Can you work these out from the model? Positions are in its coordinate system, mm. A direction names the side the tool comes from. Round coordinates to 2 decimals unless told otherwise and drop trailing zeros. Order: outer loops, then holes, each group sorted by start corner. A loop starts at its lowest first (then second) coordinate and runs counter-clockwise, first axis right, second up. Notation, with made-up numbers: (-3, 26.25) -> (10, 26.25) arc R30 cw to (10, 52.25) -> close; hole circle Ø10 at (-11, 21). An arc over 180 degrees is marked (long way). Use a Markdown table: item, result. Add a question column.
Q1. If we section it at A-A on x = 45: List the corners of the cut face in (y, z) for me.
Q2. I need wall thicknesses on line 1 along X through (y, z) = (73, 5.25); line 2 along Y through (x, z) = (161.5, 5); line 3 along Y through (x, z) = (30.5, 9.75). Which ranges of each line are inside material? Lowest first, please. Write a range as [from, to].
Q3. If we section it at B-B on z = 7: Give the number of separate pieces and of enclosed holes in the cut face, plus the area to 3 significant figures.
Q4. For faces 1 (the face through (245.316, 106, 5)), 2 (the face through (39, 37.988, 5)), 3 (the face through (260, 257.988, 5)), which set-ups out of +Z, -Z, +X, -X, +Y, -Y let a thin tool reach every point of the face, with its end or its side?
Q5. I'm going to push flat-ended pins straight in: pin 1 Ø6.5 at (x, y) = (129.47, 147.99) entering from -Z; pin 2 Ø3 at (x, z) = (250, 6) entering from +Y. Where does each tip first touch, or does it pass through?
Q6. We'd pull the mould along X, two halves only. Please class faces 4 (the face through (79.971, 18, 5)), 5 (the face through (148, 150, 0)), 6 (the face through (26.971, 234, 5)): +X half, -X half, draft (parallel to the pull), parting line (faces both ways), or undercut.
```python
from build123d import *

# Parameters (mm, degrees)
SKETCH_1_R      = 2.5
SKETCH_1_R_2    = 2
SKETCH_1_W      = 4.718060626
SKETCH_1_H      = 12.511006694
SKETCH_1_W_2    = 4.554527511
SKETCH_1_H_2    = 11.281053154
SKETCH_1_H_3    = 12.511006695
SKETCH_1_H_4    = 11.281053155
EXTRUDE_1_DEPTH = 10


with BuildPart() as part:
    # 草图1 → 凸台-拉伸1 (new body)
    with BuildSketch(Plane.XY):
        with BuildLine():
            ThreePointArc((79.970680431, 2.987579423), (81.435146525, -0.547954483), (84.970680431, -2.012420577))
            Line((84.970680431, -2.012420577), (214.970680431, -2.012420577))
            ThreePointArc((214.970680431, -2.012420577), (218.506214337, -0.547954483), (219.970680431, 2.987579423))
            Line((219.970680431, 2.987579423), (219.970680431, 32.987579423))
            ThreePointArc((219.970680431, 32.987579423), (221.435146525, 36.523113329), (224.970680431, 37.987579423))
            Line((224.970680431, 37.987579423), (294.970680431, 37.987579423))
            ThreePointArc((294.970680431, 37.987579423), (298.506214337, 39.452045517), (299.970680431, 42.987579423))
            Line((299.970680431, 42.987579423), (299.970680431, 252.987579423))
            ThreePointArc((299.970680431, 252.987579423), (298.506214337, 256.523113329), (294.970680431, 257.987579423))
            Line((294.970680431, 257.987579423), (224.970680431, 257.987579423))
            ThreePointArc((224.970680431, 257.987579423), (221.435146525, 259.452045517), (219.970680431, 262.987579423))
            Line((219.970680431, 262.987579423), (219.970680431, 292.987579423))
            ThreePointArc((219.970680431, 292.987579423), (218.506214337, 296.523113329), (214.970680431, 297.987579423))
            Line((214.970680431, 297.987579423), (84.970680431, 297.987579423))
            ThreePointArc((84.970680431, 297.987579423), (81.435146525, 296.523113329), (79.970680431, 292.987579423))
            Line((79.970680431, 292.987579423), (79.970680431, 262.987579423))
            ThreePointArc((79.970680431, 262.987579423), (78.506214337, 259.452045517), (74.970680431, 257.987579423))
            Line((74.970680431, 257.987579423), (4.970680431, 257.987579423))
            ThreePointArc((4.970680431, 257.987579423), (1.435146525, 256.523113329), (-0.029319569, 252.987579423))
            Line((-0.029319569, 252.987579423), (-0.029319569, 42.987579423))
            ThreePointArc((-0.029319569, 42.987579423), (1.435146525, 39.452045517), (4.970680431, 37.987579423))
            Line((4.970680431, 37.987579423), (74.970680431, 37.987579423))
            ThreePointArc((74.970680431, 37.987579423), (78.506214337, 36.523113329), (79.970680431, 32.987579423))
            Line((79.970680431, 32.987579423), (79.970680431, 2.987579423))
        make_face()
        with Locations((9.970680431, 47.987579423)):
            Circle(SKETCH_1_R, mode=Mode.SUBTRACT)
        with BuildLine():
            ThreePointArc((22.970680431, 70.487579423), (24.970680431, 72.487579423), (26.970680431, 70.487579423))
            Line((26.970680431, 70.487579423), (26.970680431, 52.987579423))
            ThreePointArc((26.970680431, 52.987579423), (24.970680431, 50.987579423), (22.970680431, 52.987579423))
            Line((22.970680431, 52.987579423), (22.970680431, 70.487579423))
        make_face(mode=Mode.SUBTRACT)
        with BuildLine():
            ThreePointArc((52.970680431, 70.487579423), (54.970680431, 72.487579423), (56.970680431, 70.487579423))
            Line((56.970680431, 70.487579423), (56.970680431, 52.987579423))
            ThreePointArc((56.970680431, 52.987579423), (54.970680431, 50.987579423), (52.970680431, 52.987579423))
            Line((52.970680431, 52.987579423), (52.970680431, 70.487579423))
        make_face(mode=Mode.SUBTRACT)
        with BuildLine():
            ThreePointArc((76.446824756, 47.714083435), (73.446824756, 44.714083435), (70.446824756, 47.714083435))
            Line((70.446824756, 47.714083435), (70.446824756, 72.714083435))
            ThreePointArc((70.446824756, 72.714083435), (73.446824756, 75.714083435), (76.446824756, 72.714083435))
            Line((76.446824756, 72.714083435), (76.446824756, 47.714083435))
        make_face(mode=Mode.SUBTRACT)
        with Locations((30.470680431, 147.987579423)):
            Circle(SKETCH_1_R, mode=Mode.SUBTRACT)
        with Locations((79.970680431, 98.487579423)):
            Circle(SKETCH_1_R, mode=Mode.SUBTRACT)
        with Locations((129.470680431, 147.987579423)):
            Circle(SKETCH_1_R, mode=Mode.SUBTRACT)
        with BuildLine():
            Line((229.494536105, 72.714083435), (229.494536105, 47.714083435))
            ThreePointArc((229.494536105, 47.714083435), (226.494536105, 44.714083435), (223.494536105, 47.714083435))
            Line((223.494536105, 47.714083435), (223.494536105, 72.714083435))
            ThreePointArc((223.494536105, 72.714083435), (226.494536105, 75.714083435), (229.494536105, 72.714083435))
        make_face(mode=Mode.SUBTRACT)
        with BuildLine():
            ThreePointArc((242.970680431, 70.487579423), (244.970680431, 72.487579423), (246.970680431, 70.487579423))
            Line((246.970680431, 70.487579423), (246.970680431, 52.987579423))
            ThreePointArc((246.970680431, 52.987579423), (244.970680431, 50.987579423), (242.970680431, 52.987579423))
            Line((242.970680431, 52.987579423), (242.970680431, 70.487579423))
        make_face(mode=Mode.SUBTRACT)
        with Locations((289.970680431, 47.987579423)):
            Circle(SKETCH_1_R_2, mode=Mode.SUBTRACT)
        with BuildLine():
            ThreePointArc((276.970680431, 52.987579423), (274.970680431, 50.987579423), (272.970680431, 52.987579423))
            Line((272.970680431, 52.987579423), (272.970680431, 70.487579423))
            ThreePointArc((272.970680431, 70.487579423), (274.970680431, 72.487579423), (276.970680431, 70.487579423))
            Line((276.970680431, 70.487579423), (276.970680431, 52.987579423))
        make_face(mode=Mode.SUBTRACT)
        with Locations((160.553347356, 126.301390813)):
            Circle(SKETCH_1_R_2, mode=Mode.SUBTRACT)
        with Locations((215.033347356, 126.301390813)):
            Circle(SKETCH_1_R_2, mode=Mode.SUBTRACT)
        with Locations((242.957198236, 106.410275276)):
            Rectangle(SKETCH_1_W, SKETCH_1_H, mode=Mode.SUBTRACT)
        with Locations((289.593492305, 105.795298506)):
            Rectangle(SKETCH_1_W_2, SKETCH_1_H_2, mode=Mode.SUBTRACT)
        with Locations((79.970680431, 197.487579423)):
            Circle(SKETCH_1_R, mode=Mode.SUBTRACT)
        with BuildLine():
            Line((26.970680431, 242.987579423), (26.970680431, 225.487579423))
            ThreePointArc((26.970680431, 225.487579423), (24.970680431, 223.487579423), (22.970680431, 225.487579423))
            Line((22.970680431, 225.487579423), (22.970680431, 242.987579423))
            ThreePointArc((22.970680431, 242.987579423), (24.970680431, 244.987579423), (26.970680431, 242.987579423))
        make_face(mode=Mode.SUBTRACT)
        with Locations((9.970680431, 247.987579423)):
            Circle(SKETCH_1_R, mode=Mode.SUBTRACT)
        with BuildLine():
            Line((56.970680431, 242.987579423), (56.970680431, 225.487579423))
            ThreePointArc((56.970680431, 225.487579423), (54.970680431, 223.487579423), (52.970680431, 225.487579423))
            Line((52.970680431, 225.487579423), (52.970680431, 242.987579423))
            ThreePointArc((52.970680431, 242.987579423), (54.970680431, 244.987579423), (56.970680431, 242.987579423))
        make_face(mode=Mode.SUBTRACT)
        with BuildLine():
            Line((70.446824756, 223.261075411), (70.446824756, 248.261075411))
            ThreePointArc((70.446824756, 248.261075411), (73.446824756, 251.261075411), (76.446824756, 248.261075411))
            Line((76.446824756, 248.261075411), (76.446824756, 223.261075411))
            ThreePointArc((76.446824756, 223.261075411), (73.446824756, 220.261075411), (70.446824756, 223.261075411))
        make_face(mode=Mode.SUBTRACT)
        with Locations((113.606281629, 236.082638095)):
            Circle(SKETCH_1_R_2, mode=Mode.SUBTRACT)
        with Locations((113.606281629, 268.082638095)):
            Circle(SKETCH_1_R_2, mode=Mode.SUBTRACT)
        with Locations((160.553347356, 187.721390813)):
            Circle(SKETCH_1_R_2, mode=Mode.SUBTRACT)
        with Locations((215.033347356, 187.721390813)):
            Circle(SKETCH_1_R_2, mode=Mode.SUBTRACT)
        with Locations((190.106281629, 220.582638095)):
            Circle(SKETCH_1_R_2, mode=Mode.SUBTRACT)
        with Locations((242.957198236, 189.56488357)):
            Rectangle(SKETCH_1_W, SKETCH_1_H_3, mode=Mode.SUBTRACT)
        with Locations((289.593492305, 190.17986034)):
            Rectangle(SKETCH_1_W_2, SKETCH_1_H_4, mode=Mode.SUBTRACT)
        with Locations((189.606281629, 283.582638095)):
            Circle(SKETCH_1_R_2, mode=Mode.SUBTRACT)
        with BuildLine():
            ThreePointArc((223.494536105, 248.261075411), (226.494536105, 251.261075411), (229.494536105, 248.261075411))
            Line((229.494536105, 248.261075411), (229.494536105, 223.261075411))
            ThreePointArc((229.494536105, 223.261075411), (226.494536105, 220.261075411), (223.494536105, 223.261075411))
            Line((223.494536105, 223.261075411), (223.494536105, 248.261075411))
        make_face(mode=Mode.SUBTRACT)
        with BuildLine():
            Line((246.970680431, 242.987579423), (246.970680431, 225.487579423))
            ThreePointArc((246.970680431, 225.487579423), (244.970680431, 223.487579423), (242.970680431, 225.487579423))
            Line((242.970680431, 225.487579423), (242.970680431, 242.987579423))
            ThreePointArc((242.970680431, 242.987579423), (244.970680431, 244.987579423), (246.970680431, 242.987579423))
        make_face(mode=Mode.SUBTRACT)
        with BuildLine():
            Line((272.970680431, 225.487579423), (272.970680431, 242.987579423))
            ThreePointArc((272.970680431, 242.987579423), (274.970680431, 244.987579423), (276.970680431, 242.987579423))
            Line((276.970680431, 242.987579423), (276.970680431, 225.487579423))
            ThreePointArc((276.970680431, 225.487579423), (274.970680431, 223.487579423), (272.970680431, 225.487579423))
        make_face(mode=Mode.SUBTRACT)
        with Locations((289.970680431, 247.987579423)):
            Circle(SKETCH_1_R, mode=Mode.SUBTRACT)
    extrude(amount=EXTRUDE_1_DEPTH)


solid = part.part
```
Answer below:
| question | item | result |
|---|---|---|
| 1 | outline | (37.99, 0) -> (257.99, 0) -> (257.99, 10) -> (37.99, 10) -> close |
| 2 | line 1 | [-0.03, 70.46], [76.43, 223.51], [229.48, 299.97] |
| 2 | line 2 | [-2.01, 124.54], [128.06, 185.96], [189.48, 297.99] |
| 2 | line 3 | [37.99, 145.49], [150.49, 257.99] |
| 3 | separate pieces | 1 |
| 3 | enclosed holes | 32 |
| 3 | area | 75,300 mm² |
| 4 | face 1 | +Z, -Z |
| 4 | face 2 | +Z, -Z, -X, -Y |
| 4 | face 3 | +Z, -Z, +X, +Y |
| 5 | pin 1 | z = 0 |
| 5 | pin 2 | y = 257.99 |
| 6 | face 4 | -X half |
| 6 | face 5 | draft |
| 6 | face 6 | undercut |
